The drawing under review shows one solid part. Ordinate dimensions are in mm from its lowest x, y, z. Round coordinates to 2 decimals unless told otherwise and drop trailing zeros. Loops run counter-clockwise (first coordinate to the right, second up) from the corner with the lowest first, then second, coordinate; pieces in that order, holes last. Notation, with made-up numbers: (-18, 45) - (15, 45) arc R24 cw to (15, 73) - close; hole circle Ø11 at (-19, -32). An arc over 180 degrees is marked (long way). Answer as CSV lines item,"result".
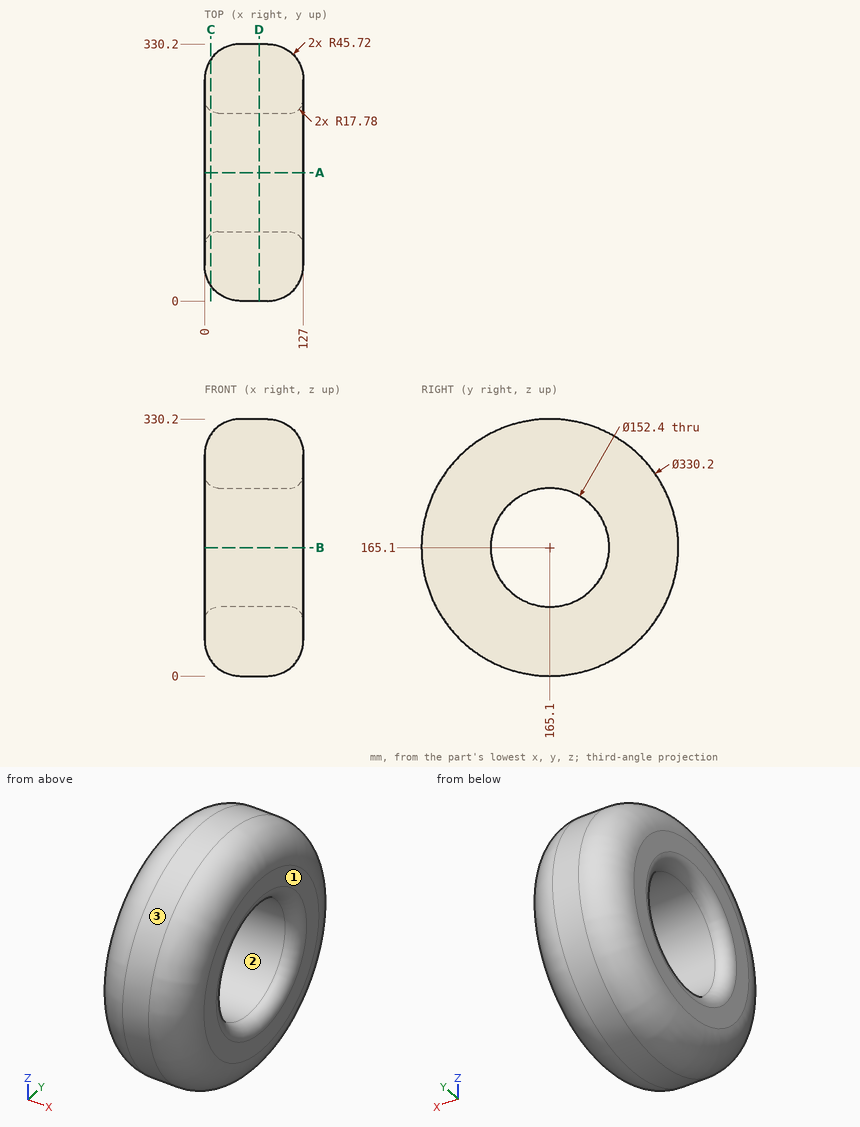
1. Take a section at C-C (x = 8). State the section outline as (y, z) points, plus the area to 3 significant figures.
Numbers:
outline,"circle Ø290.43 at (165.1, 165.1); hole circle Ø158.26 at (165.1, 165.1)"
area,"46,600 mm²"
2. Draft analysis for pull direction Z (two halves, no side actions). For the marked faces 1, 2 and 3, state which applies: +Z half, -Z half, draft (parallel to the pull), parting line (faces both ways), or undercut.
Numbers:
face 1,"draft"
face 2,"undercut"
face 3,"parting line"
3. Wall thickness on probe 1 along Y at (x, z) = (65, 165); probe 2 along X at (y, z) = (267, 102); probe 3 along Y at (x, z) = (39.5, 116): over which ranges is each line inside the solid? List them lowest first.
Numbers:
probe 1,"y = 0 to 88.9, 241.3 to 330.2"
probe 2,"x = 0 to 127"
probe 3,"y = 7.92 to 106.83, 223.37 to 322.28"
4. Take a section at D-D (x = 70). State the section outline as (y, z) points.
Numbers:
outline,"circle Ø330.2 at (165.1, 165.1); hole circle Ø152.4 at (165.1, 165.1)"
5. Take a section at A-A (y = 165.1). State the section outline as (x, z) points.
Numbers:
outline,"(0, 45.72) arc R45.72 ccw to (45.72, 0) - (81.28, 0) arc R45.72 ccw to (127, 45.72) - (127, 71.12) arc R17.78 ccw to (109.22, 88.9) - (17.78, 88.9) arc R17.78 ccw to (0, 71.12) - close; (0, 259.08) arc R17.78 ccw to (17.78, 241.3) - (109.22, 241.3) arc R17.78 ccw to (127, 259.08) - (127, 284.48) arc R45.72 ccw to (81.28, 330.2) - (45.72, 330.2) arc R45.72 ccw to (0, 284.48) - close"
6. Clearance check with flat-ended pins moving along their axes: pin 1 (4 mm diameter, centred on x = 58.5, y = 267.5, fed in from -Z); pin 2 (8 mm diameter, centred on x = 59.5, z = 195.5, fed in from +Y); pin 3 (10 mm diameter, centred on x = 78, y = 132, fed in from +Z); pin 4 (8 mm diameter, centred on y = 281, z = 162.5, fed in from -X). State where each tip first meets the part, or that it passes through.
Numbers:
pin 1,"stops at z = 34.04"
pin 2,"stops at y = 328.08"
pin 3,"stops at z = 327.79"
pin 4,"stops at x = 0"
